Check sheet for the modelled part. Datum: model origin and axes. Units: mm. A direction names the side the tool comes from. Round coordinates to 2 decimals unless told otherwise and drop trailing zeros. Order: outer loops, then holes, each group sorted by start corner. A loop starts at its lowest first (then second) coordinate and runs counter-clockwise, first axis right, second up.
from build123d import *

# Parameters (mm, degrees)
MAIN_BODY_DEPTH       = 5
SKETCH3_R             = 6.985
BEARING_CUTOUT_DEPTH  = 3
SKETCH4_R             = 1.5
TOP_MOUNT_HOLES_DEPTH = 10
SKETCH6_W             = 15
SKETCH6_H             = 10
SKETCH6_R             = 2
MOUNTING_HOLES_DEPTH  = 5
FILLET1_R             = 5


with BuildPart() as part:
    # Sketch1 → main body (new body, symmetric)
    with BuildSketch(Plane(origin=(0, 0, 0), x_dir=(1, 0, 0), z_dir=(0, 1, 0))):
        with BuildLine():
            Line((20, 0), (12.7, 0))
            Line((12.7, 0), (5.715, 0))
            ThreePointArc((5.715, 0), (0, -5.715), (-5.715, 0))
            Line((-5.715, 0), (-12.7, 0))
            Line((-12.7, 0), (-20, 0))
            Line((-20, 0), (-20, -32.5))
            Line((-20, -32.5), (20, -32.5))
            Line((20, -32.5), (20, 0))
        make_face()
    extrude(amount=MAIN_BODY_DEPTH, both=True)

    # Sketch3 → bearing cutout (cut, symmetric)
    with BuildSketch(Plane(origin=(0, 0, 0), x_dir=(1, 0, 0), z_dir=(0, 1, 0))):
        Circle(SKETCH3_R)
    extrude(amount=BEARING_CUTOUT_DEPTH, both=True, mode=Mode.SUBTRACT)

    # Sketch4 → top mount holes (cut)
    with BuildSketch(Plane(origin=(0, 0, 0), x_dir=(-1, 0, 0), z_dir=(0, 0, -1))):
        with Locations((-15, 0)):
            Circle(SKETCH4_R)
        with Locations((15, 0)):
            Circle(SKETCH4_R)
    extrude(amount=-TOP_MOUNT_HOLES_DEPTH, mode=Mode.SUBTRACT)

    # Sketch6 → mounting holes (add)
    with BuildSketch(Plane.XY.offset(32.5)):
        with Locations((-27.5, 0)):
            Rectangle(SKETCH6_W, SKETCH6_H)
        with Locations((-30, 0)):
            Circle(SKETCH6_R, mode=Mode.SUBTRACT)
        with Locations((27.5, 0)):
            Rectangle(SKETCH6_W, SKETCH6_H)
        with Locations((30, 0)):
            Circle(SKETCH6_R, mode=Mode.SUBTRACT)
    extrude(amount=-MOUNTING_HOLES_DEPTH)

    # Fillet1
    fillet1_edges = [part.edges().sort_by_distance(p)[0] for p in [
        (-20, 0, 27.5),
        (20, 0, 27.5),
    ]]
    fillet(fillet1_edges, radius=FILLET1_R)


solid = part.part
1) Sectioned sample at D-D on x = 0. Record the cut outline in (y, z) (3 decimals).
2) Gauge pin test, flat ends, axial feed: pin 1 (2 mm diameter, centred on y = 3, z = 25.5, fed in from +X); pin 2 (5 mm diameter, centred on x = -28, y = -2, fed in from -Z); pin 3 (4 mm diameter, centred on y = -3, z = 23.5, fed in from +X). Record the tip position at first contact, or that the pin passes through.
3) Sectioned sample at A-A on y = 0. Record the cut outline in (x, z) (3 decimals), and give its area (3 significant figures).
4) Set-up check for faces 1 (the face through (-13, 0, 0)), 2 (the face through (-28.092, 0.601, 30.035)), 3 (the face through (32.2, 0.1, 27.5)), 4 (the face through (-13.5, 0.07, 4.93)), 5 (the face through (-20, 0, 11)): record each of +Z, -Z, +X, -X, +Y, -Y from which the full face is reachable in a straight line by a thin tool's end or side.
5) Sectioned sample at B-B on x = -30. Record the cut outline in (y, z), and give its area (3 significant figures).
6) Sectioned sample at C-C on z = 29.5. Record the cut outline in (x, y).
7) Draft check along Y on faces 6 (the face through (0, -5, 20)), 7 (the face through (35, 0, 30)), 8 (the face through (16.5, 0.07, 4.93)), 9 (the face through (0, 3, 6)). Enter one of: pulls with the +Y half, pulls with the -Y half, needs draft (parallel to the pull), parting line crosses it, or undercut.
8) Scan lines: line 1 (Y direction, x = -30, z = 29); line 2 (Y direction, x = -15, z = 3); line 3 (X direction, y = 1, z = 4). Record each from-to range of solid material in increasing order.
Values found:
1. outline: (-5, 5.715) - (-3, 5.715) - (-3, 6.985) - (3, 6.985) - (3, 5.715) - (5, 5.715) - (5, 32.5) - (-5, 32.5) - close
2. pin 1: stops at x = 22
2. pin 2: stops at z = 27.5
2. pin 3: stops at x = 21
3. outline: (-35, 27.5) - (-32, 27.5) - (-32, 32.5) - (-35, 32.5) - close; (-28, 27.5) - (-25, 27.5) arc R5 cw to (-20, 22.5) - (-20, 0) - (-16.5, 0) - (-16.5, 10) - (-13.5, 10) - (-13.5, 0) - (-6.985, 0) arc R6.985 cw to (6.985, 0) - (13.5, 0) - (13.5, 10) - (16.5, 10) - (16.5, 0) - (20, 0) - (20, 22.5) arc R5 cw to (25, 27.5) - (28, 27.5) - (28, 32.5) - (-28, 32.5) - close; (32, 27.5) - (35, 27.5) - (35, 32.5) - (32, 32.5) - close
3. area: 1,280 mm2
4. face 1: -Z, +X, -X, +Y, -Y
4. face 2: +Z, -Z
4. face 3: -Z, +X, +Y, -Y
4. face 4: -Z
4. face 5: -Z, -X, +Y, -Y
5. outline: (-5, 27.5) - (-2, 27.5) - (-2, 32.5) - (-5, 32.5) - close; (2, 27.5) - (5, 27.5) - (5, 32.5) - (2, 32.5) - close
5. area: 30.0 mm2
6. outline: (-35, -5) - (35, -5) - (35, 5) - (-35, 5) - close; hole circle Ø4 at (-30, 0); hole circle Ø4 at (30, 0)
7. face 6: pulls with the -Y half
7. face 7: needs draft
7. face 8: undercut
7. face 9: undercut
8. line 1: y = -5 to -2, 2 to 5
8. line 2: y = -5 to -1.5, 1.5 to 5
8. line 3: x = -20 to -16.12, -13.88 to -5.73, 5.73 to 13.88, 16.12 to 20
